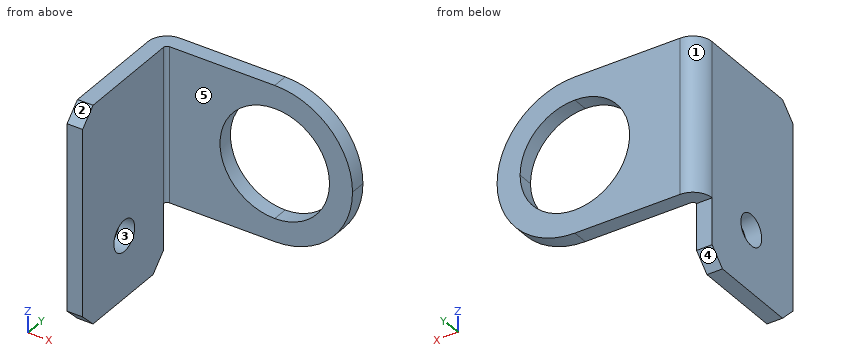
from build123d import *

# Parameters (mm, degrees)
BASE_FLANGE1_DEPTH  = 15.875
CUT_EXTRUDE1_DEPTH  = 51.201157855
SKETCH8_W           = 12.7
SKETCH8_H           = 24.6634
TAB1_DEPTH          = 3.175
SKETCH7_R           = 3.175
CUT_EXTRUDE2_DEPTH  = 54.975
BREAK_CORNER1_START = -3.175
BREAK_CORNER1_DEPTH = 3.175


# Read off the part's stored shape, not the designer's step: Break-Corner1
# Sheet-metal steps are written as plain solids
with BuildPart() as part:
    # Sketch1 → Base-Flange1 (new, symmetric)
    with BuildSketch(Plane.XY):
        with BuildLine():
            Line((0, -25.4), (0, -0.7366))
            ThreePointArc((0, -0.7366), (0.215745145, -0.215745145), (0.7366, 0))
            Line((0.7366, 0), (38.1, 0))
            Line((38.1, 0), (38.1, 3.175))
            Line((38.1, 3.175), (0.7366, 3.175))
            ThreePointArc((0.7366, 3.175), (-2.029318885, 2.029318885), (-3.175, -0.7366))
            Line((-3.175, -0.7366), (-3.175, -25.4))
            Line((-3.175, -25.4), (0, -25.4))
        make_face()
    extrude(amount=BASE_FLANGE1_DEPTH, both=True)

    # Sketch6 → Cut-Extrude1 (cut, through all)
    with BuildSketch(Plane(origin=(0, 3.175, 0), x_dir=(1, 0, 0), z_dir=(0, 1, 0))):
        with BuildLine():
            Line((38.1, -15.875), (38.1, -6.7e-08))
            ThreePointArc((38.1, -6.7e-08), (33.450320128, -11.225320175), (22.225, -15.875))
            Line((22.225, -15.875), (38.1, -15.875))
        make_face()
        with BuildLine():
            Line((38.1, 15.875), (22.225, 15.875))
            ThreePointArc((22.225, 15.875), (33.450320175, 11.225320128), (38.1, -6.7e-08))
            Line((38.1, -6.7e-08), (38.1, 15.875))
        make_face()
        with BuildLine():
            ThreePointArc((33.401, 0), (30.127625387, 7.902625387), (22.225, 11.176))
            Line((22.225, 11.176), (22.225, -11.176))
            ThreePointArc((22.225, -11.176), (30.127625387, -7.902625387), (33.401, 0))
        make_face()
        with BuildLine():
            Line((22.225, -11.176), (22.225, 11.176))
            ThreePointArc((22.225, 11.176), (11.049, 0), (22.225, -11.176))
        make_face()
    extrude(amount=-CUT_EXTRUDE1_DEPTH, mode=Mode.SUBTRACT)

    # Sketch8 → Tab1 (add)
    with BuildSketch(Plane(origin=(0, 0, 0), x_dir=(0, 0, -1), z_dir=(1, 0, 0))):
        with Locations((22.225, -13.0683)):
            Rectangle(SKETCH8_W, SKETCH8_H)
    extrude(amount=-TAB1_DEPTH)

    # Sketch7 → Cut-Extrude2 (cut, through all)
    with BuildSketch(Plane(origin=(0, 0, 0), x_dir=(0, 0, -1), z_dir=(1, 0, 0))):
        with Locations((15.875, -12.7)):
            Circle(SKETCH7_R)
    extrude(amount=-CUT_EXTRUDE2_DEPTH, mode=Mode.SUBTRACT)

    # Break-Corner1 outline → Break-Corner1 (cut)
    with BuildSketch(Plane.YZ.offset(BREAK_CORNER1_START)):
        Polygon((-25.4, -28.575), (-22.225, -28.575), (-25.4, -25.4), align=None)
        Polygon((-25.4, 15.875), (-25.4, 12.7), (-22.225, 15.875), align=None)
        Polygon((-0.7366, -25.4), (-3.9116, -28.575), (-0.7366, -28.575), align=None)
    extrude(amount=BREAK_CORNER1_DEPTH, mode=Mode.SUBTRACT)


solid = part.part
Source: CAD feature listing. Evaluate the final solid. Frame: model axes, mm. Face numbers are marked on the shaded views. A direction names the side the tool comes from. Coordinates: 2 decimals unless noted, no trailing zeros. Order: outer loops, then holes, each group sorted by start corner. A loop starts at its lowest first (then second) coordinate and runs counter-clockwise, first axis right, second up. Notation, with made-up numbers: M 19.25,-23 L 27.25,-23 A33 cw 27.25,13 Z; hole C -10,-27 d3. An arc over 180 degrees is marked long. Write each question's results on one line, items separated by ' | '. Start each with the question number.
1. Draft query along Y for the marked faces 1, 2 and 3. Return one class per face: +Y half, -Y half, draft (parallel to the pull), parting line (faces both ways), or undercut.
2. Reachability of the marked faces 4 and 5 from +Z, -Z, +X, -X, +Y, -Y: full face, straight path, thin tool, end or side. Return the list, or none.
3. Section C-C, the plane x = 30.5. Return the cut outline in (y, z) (3 decimals).
4. Section D-D, the plane y = -23.5. Return the cut outline in (x, z) (3 decimals).
5. Section A-A, the plane y = -12.7. Return the cut outline in (x, z) (3 decimals).
6. Section B-B, the plane z = -14. Return the cut outline in (x, y) (3 decimals), then the cut area to 3 significant figures.
7. Pin query (flat end, axial travel): pin 1 (2 mm diameter, centred on x = 15.5, y = 0.5, fed in from -Z) (3 decimals); pin 2 (1 mm diameter, centred on y = -2, z = -23, fed in from +X); pin 3 (1 mm diameter, centred on x = -1.5, z = -20, fed in from +Y); pin 4 (8 mm diameter, centred on x = 30, z = -1.5, fed in from +Y) (3 decimals). Return the tip coordinate at first contact, or that it passes through.
8. Material intervals for L1, parallel to X at y = -8.25, z = -19.5 (3 decimals); L2, parallel to Y at x = 4.5, z = 8 (3 decimals), sorted ascending.
Solution:
1) face 1: +Y half | face 2: -Y half | face 3: undercut
2) face 4: -Z, +X, -X, +Y | face 5: +Z, -Z, +X, -Y
3) outline: M 0,-13.548 L 3.175,-13.548 L 3.175,-7.512 L 0,-7.512 Z; M 0,7.512 L 3.175,7.512 L 3.175,13.548 L 0,13.548 Z
4) outline: M -3.175,-27.3 L 0,-27.3 L 0,14.6 L -3.175,14.6 Z
5) outline: M -3.175,-28.575 L 0,-28.575 L 0,-19.05 L -3.175,-19.05 Z; M -3.175,-12.7 L 0,-12.7 L 0,15.875 L -3.175,15.875 Z
6) outline: M -3.175,-25.4 L 0,-25.4 L 0,-15.262 L -3.175,-15.262 Z; M -3.175,-10.138 L 0,-10.138 L 0,-0.737 A0.737 cw 0.737,0 L 29.709,0 L 29.709,3.175 L 0.737,3.175 A3.912 ccw -3.175,-0.737 Z | area: 166 mm²
7) pin 1: z = -15.875 | pin 2: x = 0 | pin 3: y = -0.74 | pin 4: y = 3.175
8) L1: -3.175 to 0 | L2: 0 to 3.175
